Can you work these out from the model? Positions are in its coordinate system, mm. Coordinates: 2 decimals unless noted, no trailing zeros. Loops run counter-clockwise (first coordinate to the right, second up) from the corner with the lowest first, then second, coordinate; pieces in that order, holes last. Notation, with made-up numbers: (-37.5, 19.5) -> (-25.5, 19.5) arc R32 cw to (-25.5, 48.5) -> close; hole circle Ø11 at (84.5, 58). An arc over 180 degrees is marked (long way). Use one line per item in the form item = value. Start each with the question number.
(1) Imagine slicing it at D-D (x = 27.5). List the corners of the cut face in (y, z) for me.
(2) Imagine slicing it at A-A (y = 5.1). List the corners of the cut face in (x, z) for me (3 decimals), plus the area to 3 significant figures.
(3) I'm going to push flat-ended pins straight in: pin 1 (5 mm diameter, centred on x = 0, z = 0, fed in from -Y); pin 2 (1 mm diameter, centred on y = 4, z = 64.5, fed in from +X); pin 3 (1 mm diameter, centred on x = 8.5, y = 1.5, fed in from -Z). Where does each tip first touch, or does it pass through?
(4) Imagine slicing it at B-B (x = -4.5). List the corners of the cut face in (y, z) for me, plus the area to 3 significant figures.
(5) Thinking about a two-plate mould opening in Z: for faces 1 (the flat face through (-1, 0, -26)), 2 (the flat face through (45.057, 2.958, 13.363)), 3 (the cylindrical face through (5.5, 3, 99.9)), which applies, released by +Z, released by -Z, zero draft, split by the parting line, or undercut?
(6) Imagine slicing it at C-C (z = 61). List the corners of the cut face in (x, y) for me, plus the area to 3 significant figures.
(7) I need wall thicknesses on line 1 (Z direction, x = -0.5, y = 4.7); line 2 (X direction, y = 2.35, z = 0); line 3 (Z direction, x = 22, y = 0.7). Which ranges of each line are inside material? Lowest first, please. Write a range as [from, to].
```python
from build123d import *

# Parameters (mm, degrees)
SKETCH1_R           = 1.5
BOSS_EXTRUDE1_DEPTH = 6
CUT_EXTRUDE1_START  = -10
CUT_EXTRUDE1_DEPTH  = 10


with BuildPart() as part:
    # Sketch1 → Boss-Extrude1 (new body)
    # profile 1 of 3: a face of its own
    with BuildSketch(Plane(origin=(0, 0, 0), x_dir=(1, 0, 0), z_dir=(0, 1, 0))):
        with BuildLine():
            ThreePointArc((110, 0), (97.61406367, 50.709906072), (63.245553203, 90))
            Line((63.245553203, 90), (1.5, 90))
            ThreePointArc((1.5, 90), (0, 88.5), (-1.5, 90))
            Line((-1.5, 90), (-63.245553203, 90))
            ThreePointArc((-63.245553203, 90), (-109.405676864, 11.419188675), (-80.467384697, -75))
            Line((-80.467384697, -75), (-25.5, -75))
            ThreePointArc((-25.5, -75), (0, -49.5), (25.5, -75))
            Line((25.5, -75), (80.467384697, -75))
            ThreePointArc((80.467384697, -75), (102.350897203, -40.302528973), (110, 0))
        make_face()
        with Locations(Location((0, 0, 0), (0, 0, 270))):
            Circle(SKETCH1_R, mode=Mode.SUBTRACT)
    # profile 2 of 3: a face of its own
    with BuildSketch(Plane(origin=(0, 0, 0), x_dir=(1, 0, 0), z_dir=(0, 1, 0))):
        with BuildLine():
            ThreePointArc((-80.467384697, -75), (0, -110), (80.467384697, -75))
            Line((80.467384697, -75), (25.5, -75))
            ThreePointArc((25.5, -75), (0, -100.5), (-25.5, -75))
            Line((-25.5, -75), (-80.467384697, -75))
        make_face()
    # profile 3 of 3: a face of its own
    with BuildSketch(Plane(origin=(0, 0, 0), x_dir=(1, 0, 0), z_dir=(0, 1, 0))):
        with BuildLine():
            Line((1.5, 90), (63.245553203, 90))
            ThreePointArc((63.245553203, 90), (0, 110), (-63.245553203, 90))
            Line((-63.245553203, 90), (-1.5, 90))
            ThreePointArc((-1.5, 90), (0, 91.5), (1.5, 90))
        make_face()
    extrude(amount=BOSS_EXTRUDE1_DEPTH)

    # Sketch2 → Cut-Extrude1 (cut)
    with BuildSketch(Plane(origin=(0, 6, 0), x_dir=(1, 0, 0), z_dir=(0, 1, 0)).offset(CUT_EXTRUDE1_START)):
        with BuildLine():
            Line((54.350525887, 46.572643608), (35.5, -75))
            ThreePointArc((35.5, -75), (27.52606276, -97.417980929), (7.18642992, -109.765))
            ThreePointArc((7.18642992, -109.765), (80.282337071, -75.198047544), (110, 0))
            ThreePointArc((110, 0), (77.781745816, 77.781746045), (-3.23e-07, 110))
            ThreePointArc((-3.23e-07, 110), (38.890872851, 93.890873079), (55, 55))
            ThreePointArc((55, 55), (54.837391093, 50.773827015), (54.350525887, 46.572643608))
        make_face()
        with BuildLine():
            ThreePointArc((-7.18642992, -109.765), (-27.52606276, -97.417980929), (-35.5, -75))
            Line((-35.5, -75), (-54.350525887, 46.572643608))
            ThreePointArc((-54.350525887, 46.572643608), (-41.764246786, 90.787535406), (-3.23e-07, 110))
            ThreePointArc((-3.23e-07, 110), (-109.941234308, 3.595135441), (-7.18642992, -109.765))
        make_face()
    extrude(amount=CUT_EXTRUDE1_DEPTH, mode=Mode.SUBTRACT)


solid = part.part
```
Worked out:
q1.outline = (0, -102.63) -> (6, -102.63) -> (6, 97.45) -> (0, 97.45) -> close
q2.outline = (-54.351, -46.573) arc R55 ccw (long way) to (54.351, -46.573) -> (35.5, 75) arc R35.5 ccw to (7.186, 109.765) arc R110 ccw to (-7.186, 109.765) arc R35.5 ccw to (-35.5, 75) -> close; hole circle Ø51 at (0, 75); hole circle Ø3 at (0, -90); hole circle Ø3 at (0, 0)
q2.area = 16,500 mm2
q3.pin_1 = 0
q3.pin_2 = 37.21
q3.pin_3 = -109.42
q4.outline = (0, -109.82) -> (6, -109.82) -> (6, 49.9) -> (0, 49.9) -> close; (0, 100.1) -> (6, 100.1) -> (6, 109.91) -> (0, 109.91) -> close
q4.area = 1,020 mm2
q5.face_1 = zero draft
q5.face_2 = released by +Z
q5.face_3 = undercut
q6.outline = (-37.67, 0) -> (-21.31, 0) -> (-21.31, 6) -> (-37.67, 6) -> close; (21.31, 0) -> (37.67, 0) -> (37.67, 6) -> (21.31, 6) -> close
q6.area = 196 mm2
q7.line_1 = [-110, -91.41], [-88.59, -1.41], [1.41, 49.5], [100.5, 110]
q7.line_2 = [-47.13, -1.5], [1.5, 47.13]
q7.line_3 = [-105.41, 62.11], [87.89, 102.86]
